For this review, use the dimensioned drawing (mm, ordinates from the lowest corner) and the shaded views. A direction names the side the tool comes from. Coordinates: 2 decimals unless noted, no trailing zeros. Write each loop counter-clockwise with the first axis right and the second up, starting at its lowest first coordinate (ties: lowest second). Pieces come first, ordered by that corner, then holes. Notation, with made-up numbers: (-36, -26) -> (-3, -26) arc R17 cw to (-3, 2) -> close; hole circle Ø4 at (7, 76.25). An arc over 180 degrees is marked (long way). Return JSON: item names as keys, results as strings. Group by question number.
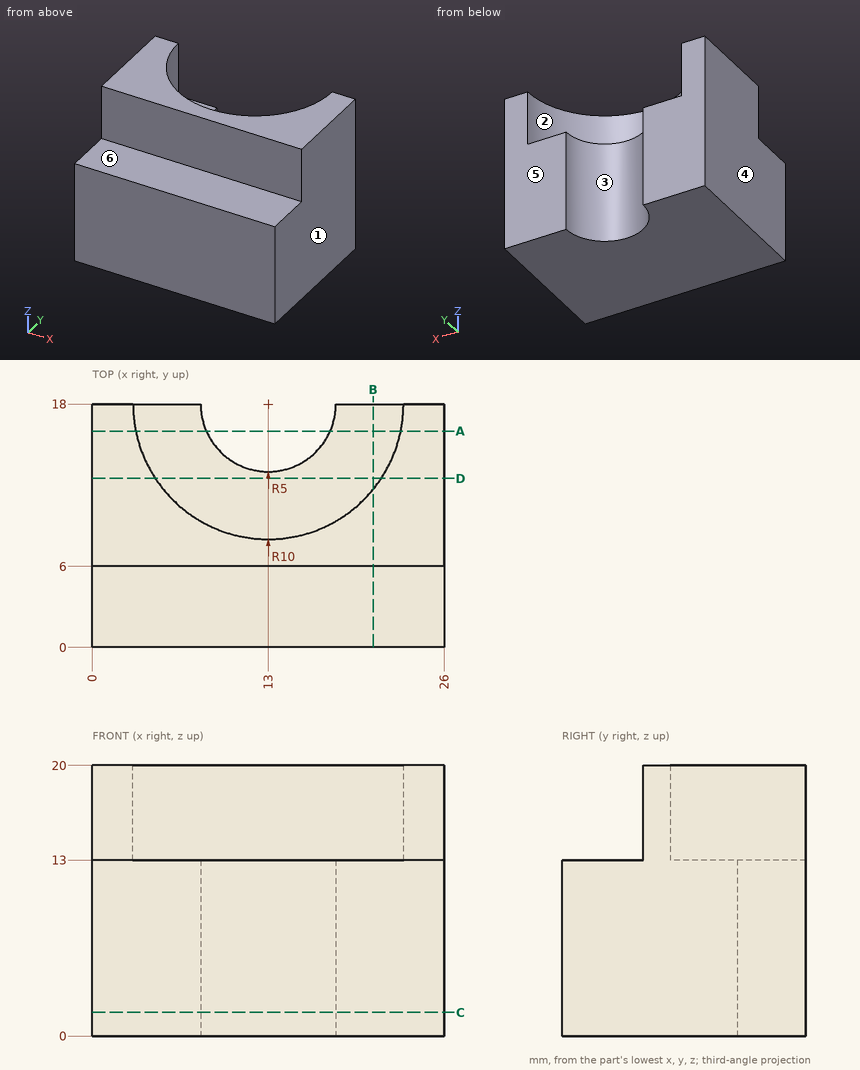
Q1. We need section C-C on z = 1.75. Write out the cut boundary in (x, y), plus the area to 3 significant figures.
Q2. We need section D-D on y = 12.5. Write out the cut boundary in (x, z), plus the area to 3 significant figures.
Q3. We need section A-A on y = 16. Write out the cut boundary in (x, z).
Q4. Wall thickness on L1, parallel to Z at x = 7.25, y = 4.5; L2, parallel to X at y = 15.75, z = 4.75; L3, parallel to X at y = 10, z = 14.5: over which ranges is each line inside the solid? List them lowest first.
Q5. We need section B-B on x = 20.75. Write out the cut boundary in (y, z).
Q6. For the marked faces 5 and 6, list the 3-axis set-ups (+Z, -Z, +X, -X, +Y, -Y) from which the entire face can be reached by the end or side of a thin tool; tool diameter is ignored.
Q7. For P1, Ø3, axis at x = 9, y = 15, coming from the +Z side; P2, Ø1.5, axis at x = 12.5, z = 15.5, coming from the -Y side, all flat-tipped, find the tip position at first contact; note any pin that passes through.
Q8. The part is to be moulded in two halves that separate along X. For the marked faces 1, 2, 3 and 4, say which applies: +X half, -X half, draft (parallel to the pull), parting line (faces both ways), or undercut.
Findings below:
{
 "1": {"outline": "(0, 0) -> (26, 0) -> (26, 18) -> (18, 18) arc R5 cw to (8, 18) -> (0, 18) -> close", "area": "429 mm^2"},
 "2": {"outline": "(0, 0) -> (26, 0) -> (26, 20) -> (21.35, 20) -> (21.35, 13) -> (4.65, 13) -> (4.65, 20) -> (0, 20) -> close", "area": "403 mm^2"},
 "3": {"outline": "(0, 0) -> (8.42, 0) -> (8.42, 13) -> (3.2, 13) -> (3.2, 20) -> (0, 20) -> close; (17.58, 0) -> (26, 0) -> (26, 20) -> (22.8, 20) -> (22.8, 13) -> (17.58, 13) -> close"},
 "4": {"L1": "z = 0 to 13", "L2": "x = 0 to 8.53, 17.47 to 26", "L3": "x = 0 to 7, 19 to 26"},
 "5": {"outline": "(0, 0) -> (18, 0) -> (18, 13) -> (11.68, 13) -> (11.68, 20) -> (6, 20) -> (6, 13) -> (0, 13) -> close"},
 "6": {"face 5": "+Z, -Z, +X, -X, +Y", "face 6": "+Z, +X, -X, -Y"},
 "7": {"P1": "stops at z = 13", "P2": "stops at y = 6"},
 "8": {"face 1": "+X half", "face 2": "undercut", "face 3": "undercut", "face 4": "-X half"}
}
